Part model, mm, in its own coordinate system. A direction names the side the tool comes from. Give positions to 0.01 mm unless a question says otherwise; leave off trailing zeros. Write each loop counter-clockwise with the first axis right and the second up, starting at its lowest first coordinate (ties: lowest second). Pieces come first, ordered by that corner, then holes. Notation, with made-up numbers: M 75,66.25 L 127,66.25 A20 ccw 127,77.25 Z; hole C 9,62.25 d1. An arc over 180 degrees is marked long. Use CSV: the item, a comma, the result in double quotes. Start each with the question number.
Item 1: Drill centre lines: line 1 (Y direction, x = 5.15, z = 3.75); line 2 (Y direction, x = 5.15, z = 1.4); line 3 (Y direction, x = 4.5, z = 11). Where is each one in solid material? Low to high. Write a range as [from, to].
Item 2: Cut at C-C (x = 5.15). List the corners of the cut face in (y, z).
Item 3: Pin check, flat tips, straight feed: pin 1 (1.7 mm diameter, centred on x = 5.5, z = 3, fed in from -Y); pin 2 (2.5 mm diameter, centred on x = 5.15, y = 3.75, fed in from +Z); pin 3 (1 mm diameter, centred on x = 8, z = 9, fed in from -Y); pin 4 (5 mm diameter, centred on x = 5, y = 4, fed in from +Z). Stop position of each tip, or through.
Item 4: Cut at A-A (z = 8.5). List the corners of the cut face in (x, y), then the cut area to 3 significant figures.
Item 5: Which spindle directions (+Z, -Z, +X, -X, +Y, -Y) get a long thin tool onto all of the face, cutting with end or side? Do faces 1 (the flat face through (5, 7.35, 9)), 2 (the flat face through (5, 25.5, 3)), 3 (the flat face through (0.15, 30, -4)), 4 (the flat face through (5, 11.85, 9)). Say none if no direction does.
Item 6: Cut at D-D (x = 7.75). List the corners of the cut face in (y, z), then the cut area to 3 significant figures.
Item 7: Mould opens along X. For faces 5 (the flat face through (8.3, 13.4, 4.7)), 6 (the flat face through (5, 10, 13.1)), 7 (the flat face through (2, 13.1, 4.7)), 8 (the cylindrical face through (4.955, 24.237, 2.586)) say: released by +X, released by -X, zero draft, split by the parting line, or undercut.
Item 8: Cut at B-B (y = 3.75). List the corners of the cut face in (x, z).
Autodesk Inventor part; units mm, degrees
ref_plane "YZ Plane" through (0, 0, 0) normal (1, 0, 0) x (0, 1, 0)
ref_plane "XZ Plane" through (0, 0, 0) normal (0, 1, 0) x (-1, 0, 0)
ref_plane "XY Plane" through (0, 0, 0) normal (0, 0, 1) x (1, 0, 0)
sketch "Sketch1" plane through (0, 0, 0) normal (0, 0, 1) x (1, 0, 0)
  line L0 (0, 0) -> (10.3, 0)
  line L1 (10.3, 0) -> (10.3, 33.2)
  line L2 (10.3, 33.2) -> (0, 33.2)
  line L3 (0, 33.2) -> (0, 0)
  dimension "d0" = 10.3
  dimension "d1" = 33.2
extrude "Extrusion1" add sketch "Sketch1" along normal blind 1.6
sketch "Sketch2" plane through (0, 0, 1.6) normal (0, 0, 1) x (1, 0, 0)
  line L0 (0, 0) -> (10.3, 0)
  line L1 (10.3, 0) -> (10.3, 33.2)
  line L2 (2, 25.5) -> (8.3, 25.5)
  line L3 (8.3, 25.5) -> (8.3, 1)
  line L4 (8.3, 1) -> (2, 1)
  line L5 (2, 1) -> (2, 25.5)
  dimension "d4" = 6.3
  dimension "d5" = 24.5
  dimension "d6" = 1
  dimension "d7" = 2
extrude "Extrusion2" add sketch "Sketch2" along normal blind 3.5
sketch "Sketch3" plane through (0, 0, 5.1) normal (0, 0, 1) x (1, 0, 0)
  line L0 (2, 25.5) -> (2, 1)
  line L1 (2, 1) -> (8.3, 1)
  line L2 (8.3, 1) -> (8.3, 25.5)
  line L3 (8.3, 11.85) -> (2, 11.85)
  line L4 (2, 7.35) -> (8.3, 7.35)
  line L5 (8.3, 14.65) -> (2, 14.65)
  line L6 (2, 19.15) -> (8.3, 19.15)
  point P0 (0, 0)
  dimension "d10" = 4.5
  dimension "d11" = 4.5
  dimension "d12" = 2.8
  dimension "d13" = 10.85
extrude "Extrusion3" add sketch "Sketch3" along normal blind 8 contours L6 L2 L5 L0 | L3 L2 L4 L0
sketch "Sketch4" plane through (0, 0, 0) normal (0, 0, -1) x (-1, 0, 0)
  line L0 (-10.3, 33.2) -> (0, 33.2)
  line L1 (-10.3, 0) -> (-10.3, 33.2)
  line L2 (-10.15, 32.4) -> (-0.15, 32.4)
  line L3 (-0.15, 32.4) -> (-0.15, 26.7)
  line L4 (-0.15, 26.7) -> (-10.15, 26.7)
  line L5 (-10.15, 26.7) -> (-10.15, 32.4)
  dimension "d16" = 10
  dimension "d17" = 5.7
  dimension "d18" = 0.15
  dimension "d19" = 0.8
extrude "Extrusion4" add sketch "Sketch4" along normal blind 7.3
sketch "Sketch5" plane through (0, 0, 5.1) normal (0, 0, 1) x (1, 0, 0)
  line L0 (2, 25.5) -> (2, 19.15)
  line L1 (8.3, 7.35) -> (2, 7.35)
  line L2 (2, 7.35) -> (2, 1)
  line L3 (2, 1) -> (8.3, 1)
  line L4 (8.3, 1) -> (8.3, 7.35)
  circle A0 centre (5.15, 3.75) radius 1.5
  circle A1 centre (5.15, 22.75) radius 1.5
  point P0 (0, 0)
  dimension "d22" = 3
  dimension "d23" = 19
  dimension "d24" = 3.15
  dimension "d25" = 2.75
extrude "Extrusion5" cut sketch "Sketch5" against normal up to next contours A0 | A1
properties part number "EndStopOptical"
Worked answers:
1,line 1,"y = [1, 2.25], [5.25, 21.25], [24.25, 25.5]"
1,line 2,"y = [0, 2.25], [5.25, 21.25], [24.25, 33.2]"
1,line 3,"y = [7.35, 11.85], [14.65, 19.15]"
2,outline,"M 0,0 L 2.25,0 L 2.25,5.1 L 1,5.1 L 1,1.6 L 0,1.6 Z; M 5.25,0 L 21.25,0 L 21.25,5.1 L 19.15,5.1 L 19.15,13.1 L 14.65,13.1 L 14.65,5.1 L 11.85,5.1 L 11.85,13.1 L 7.35,13.1 L 7.35,5.1 L 5.25,5.1 Z; M 24.25,0 L 26.7,0 L 26.7,-7.3 L 32.4,-7.3 L 32.4,0 L 33.2,0 L 33.2,1.6 L 25.5,1.6 L 25.5,5.1 L 24.25,5.1 Z"
3,pin 1,"stops at y = 1"
3,pin 2,"passes through"
3,pin 3,"stops at y = 7.35"
3,pin 4,"stops at z = 5.1"
4,outline,"M 2,7.35 L 8.3,7.35 L 8.3,11.85 L 2,11.85 Z; M 2,14.65 L 8.3,14.65 L 8.3,19.15 L 2,19.15 Z"
4,area,"56.7 mm^2"
5,face 1,"+Z, +X, -X, -Y"
5,face 2,"+Z, +X, -X, +Y"
5,face 3,"-Z, -X, +Y, -Y"
5,face 4,"+Z, +X, -X"
6,outline,"M 0,0 L 26.7,0 L 26.7,-7.3 L 32.4,-7.3 L 32.4,0 L 33.2,0 L 33.2,1.6 L 25.5,1.6 L 25.5,5.1 L 19.15,5.1 L 19.15,13.1 L 14.65,13.1 L 14.65,5.1 L 11.85,5.1 L 11.85,13.1 L 7.35,13.1 L 7.35,5.1 L 1,5.1 L 1,1.6 L 0,1.6 Z"
6,area,"252 mm^2"
7,face 5,"released by +X"
7,face 6,"zero draft"
7,face 7,"released by -X"
7,face 8,"undercut"
8,outline,"M 0,0 L 3.65,0 L 3.65,5.1 L 2,5.1 L 2,1.6 L 0,1.6 Z; M 6.65,0 L 10.3,0 L 10.3,1.6 L 8.3,1.6 L 8.3,5.1 L 6.65,5.1 Z"
